Check sheet for the modelled part. Datum: model origin and axes. Units: mm. A direction names the side the tool comes from. Round coordinates to 2 decimals unless told otherwise and drop trailing zeros. Loops run counter-clockwise (first coordinate to the right, second up) from the corner with the lowest first, then second, coordinate; pieces in that order, holes last. Notation, with made-up numbers: (26, -3.5) -> (42, -3.5) arc R5 ccw to (42, 2.5) -> close; hole circle Ø6 at (77.25, -18). An arc over 180 degrees is marked (long way). Return JSON: item names as keys, results as strings.
from build123d import *

# Parameters (mm, degrees)
SKETCH1_W                                            = 40
SKETCH1_H                                            = 60
BOSS_EXTRUDE1_DEPTH                                  = 41
M2_5_CLEARANCE_HOLE1_D                               = 2.9
CUT_EXTRUDE1_DEPTH                                   = 33.5
FILLET1_R                                            = 1.6
F_16_0_16_DIAMETER_HOLE2_D                           = 16
SKETCH9_R                                            = 15.5
CUT_EXTRUDE2_DEPTH                                   = 33.5
FILLET2_R                                            = 4
CUT_EXTRUDE3_DEPTH                                   = 65.660652641
CUT_EXTRUDE3_DEPTH_BACK                              = 14
SKETCH11_W                                           = 50.653597067
SKETCH11_H                                           = 53.338920101
SKETCH12_R                                           = 15.5
CUT_EXTRUDE4_DEPTH                                   = 61.185131054
FILLET3_R                                            = 4
BOSS_EXTRUDE3_DEPTH                                  = 3
CHAMFER1_SIZE                                        = 6
BOSS_EXTRUDE4_DEPTH                                  = 41
CUT_EXTRUDE5_DEPTH                                   = 67.715815216
CUT_EXTRUDE5_DEPTH_BACK                              = 67.715815216
SKETCH19_W                                           = 48.667082547
SKETCH19_H                                           = 18.204733745
CBORE_FOR_M2_5_HEX_SOCKET_HEAD_CAP_SCREW_D           = 2.9
CBORE_FOR_M2_5_HEX_SOCKET_HEAD_CAP_SCREW_CBORE_D     = 5
CBORE_FOR_M2_5_HEX_SOCKET_HEAD_CAP_SCREW_CBORE_DEPTH = 20
TAP_DRILL_FOR_M3_HELICOIL1_D                         = 3.2
TAP_DRILL_FOR_M3_HELICOIL1_DEPTH                     = 4
TAP_DRILL_FOR_M3_HELICOIL1_TIP                       = 0.96137699
TAP_DRILL_FOR_M3_HELICOIL2_D                         = 3.15
TAP_DRILL_FOR_M3_HELICOIL2_DEPTH                     = 4.5
TAP_DRILL_FOR_M3_HELICOIL2_TIP                       = 0.946355475


with BuildPart() as part:
    # Sketch1 → Boss-Extrude1 (new body)
    with BuildSketch(Plane(origin=(0, 0, 0), x_dir=(1, 0, 0), z_dir=(0, 1, 0))):
        with Locations((-20, 0)):
            Rectangle(SKETCH1_W, SKETCH1_H)
    extrude(amount=BOSS_EXTRUDE1_DEPTH)

    # M2.5 Clearance Hole1 (through all)
    with Locations(Plane(origin=(0, 41, 0), x_dir=(1, 0, 0), z_dir=(0, 1, 0))):
        with Locations((-37.3, 26), (-37.3, 4), (-37.3, -18), (-31, -25.8), (-9, -25.8), (-2.7, -18), (-2.7, 4), (-2.7, 26)):
            Hole(M2_5_CLEARANCE_HOLE1_D / 2)

    # Sketch4 → Cut-Extrude1 (cut)
    with BuildSketch(Plane(origin=(0, 41, 0), x_dir=(1, 0, 0), z_dir=(0, 1, 0))):
        Polygon((-34.6, 30), (-34.6, -19), (-30, -19), (-30, -23), (-10, -23), (-10, -19), (-5.4, -19), (-5.4, 30), align=None)
    extrude(amount=-CUT_EXTRUDE1_DEPTH, mode=Mode.SUBTRACT)

    # Fillet1
    fillet1_edges = [part.edges().sort_by_distance(p)[0] for p in [
        (-10, 24.25, 23),
        (-30, 24.25, 23),
        (-30, 24.25, 19),
        (-34.6, 24.25, 19),
        (-5.4, 24.25, 19),
        (-10, 24.25, 19),
    ]]
    fillet(fillet1_edges, radius=FILLET1_R)

    # Ø16.0 (16) Diameter Hole2 (through all)
    with Locations(Plane(origin=(0, 7.5, 0), x_dir=(1, 0, 0), z_dir=(0, 1, 0))):
        with Locations((-20, -6)):
            Hole(F_16_0_16_DIAMETER_HOLE2_D / 2)

    # Sketch9 → Cut-Extrude2 (cut)
    with BuildSketch(Plane(origin=(0, 7.5, 0), x_dir=(1, 0, 0), z_dir=(0, 1, 0))):
        with Locations((-20, -6)):
            Circle(SKETCH9_R)
    extrude(amount=CUT_EXTRUDE2_DEPTH, mode=Mode.SUBTRACT)

    # Fillet2
    fillet2_edges = [part.edges().sort_by_distance(p)[0] for p in [
        (-5.4, 24.25, 0.795194528),
        (-5.4, 24.25, 11.204805472),
        (-34.6, 24.25, 11.204805472),
        (-34.6, 24.25, 0.795194528),
    ]]
    fillet(fillet2_edges, radius=FILLET2_R)

    # Sketch11 → Cut-Extrude3 (cut, two sides: drawn at the far end of the back side and taken through both)
    with BuildSketch(Plane(origin=(0, 41, 0), x_dir=(1, 0, 0), z_dir=(0, 1, 0)).offset(-CUT_EXTRUDE3_DEPTH_BACK)):
        with Locations((-19.614312713, -11.741576857)):
            Rectangle(SKETCH11_W, SKETCH11_H)
    extrude(amount=CUT_EXTRUDE3_DEPTH + CUT_EXTRUDE3_DEPTH_BACK, mode=Mode.SUBTRACT)

    # Sketch12 → Cut-Extrude4 (cut, through all)
    with BuildSketch(Plane(origin=(0, 7.5, 0), x_dir=(1, 0, 0), z_dir=(0, 1, 0))):
        with Locations((-20, 22)):
            Circle(SKETCH12_R)
    extrude(amount=CUT_EXTRUDE4_DEPTH, mode=Mode.SUBTRACT)

    # Fillet3
    fillet3_edges = [part.edges().sort_by_distance(p)[0] for p in [
        (-34.6, 24.25, -27.204805472),
        (-5.4, 24.25, -27.204805472),
        (-34.6, 24.25, -16.795194528),
        (-5.4, 24.25, -16.795194528),
    ]]
    fillet(fillet3_edges, radius=FILLET3_R)

    # Sketch15 → Boss-Extrude3 (add)
    with BuildSketch(Plane(origin=(0, 0, -30), x_dir=(-1, 0, 0), z_dir=(0, 0, -1))):
        Polygon((40, 41), (34.6, 41), (34.6, 7.5), (5.4, 7.5), (5.4, 41), (0, 41), (0, 0), (40, 0), align=None)
    extrude(amount=BOSS_EXTRUDE3_DEPTH)

    # Chamfer1
    chamfer1_edges = [part.edges().sort_by_distance(p)[0] for p in [
        (0, 13.5, 30),
        (-40, 13.5, 30),
    ]]
    chamfer(chamfer1_edges, length=CHAMFER1_SIZE)

    # Sketch18 → Boss-Extrude4 (add)
    with BuildSketch(Plane.XZ):
        Polygon((0, 24), (0, -33), (1, -33), (1, 24.414213562), (-5.585786438, 31), (-34.414213562, 31), (-41, 24.414213562), (-41, -33), (-40, -33), (-40, 24), (-34, 30), (-6, 30), align=None)
    extrude(amount=-BOSS_EXTRUDE4_DEPTH)

    # Sketch19 → Cut-Extrude5 (cut, two sides: drawn at the far end of the back side and taken through both)
    with BuildSketch(Plane.ZY.offset(-CUT_EXTRUDE5_DEPTH_BACK)):
        with Locations((9.40565808, 36.102366872)):
            Rectangle(SKETCH19_W, SKETCH19_H)
    extrude(amount=CUT_EXTRUDE5_DEPTH + CUT_EXTRUDE5_DEPTH_BACK, mode=Mode.SUBTRACT)

    # CBORE for M2.5 Hex Socket Head Cap Screw1 (through all)
    with Locations(Plane(origin=(0, 0, 0), x_dir=(-1, 0, 0), z_dir=(0, -1, 0))):
        with Locations((2.7, 4), (37.3, 4), (37.3, -18), (31, -25.8), (9, -25.8), (2.7, -18), (2.7, 26), (37.3, 26)):
            CounterBoreHole(CBORE_FOR_M2_5_HEX_SOCKET_HEAD_CAP_SCREW_D / 2, CBORE_FOR_M2_5_HEX_SOCKET_HEAD_CAP_SCREW_CBORE_D / 2, CBORE_FOR_M2_5_HEX_SOCKET_HEAD_CAP_SCREW_CBORE_DEPTH)

    # Tap Drill for M3 Helicoil1
    with Locations(Plane(origin=(0, 0, -33), x_dir=(-1, 0, 0), z_dir=(0, 0, -1))):
        with Locations((37.8, 35), (8, 3.75), (32, 3.75), (2.2, 35)):
            Hole(TAP_DRILL_FOR_M3_HELICOIL1_D / 2, depth=TAP_DRILL_FOR_M3_HELICOIL1_DEPTH)
            with Locations((0, 0, -(TAP_DRILL_FOR_M3_HELICOIL1_DEPTH + TAP_DRILL_FOR_M3_HELICOIL1_TIP / 2))):  # 118° drill point
                Cone(0, TAP_DRILL_FOR_M3_HELICOIL1_D / 2, TAP_DRILL_FOR_M3_HELICOIL1_TIP, mode=Mode.SUBTRACT)

    # Tap Drill for M3 Helicoil2
    with Locations(Plane.ZY.offset(41)):
        with Locations((7, 6.75), (7, 13.5), (7, 20.25), (-15, 6.75), (-15, 13.5), (-15, 20.25)):
            Hole(TAP_DRILL_FOR_M3_HELICOIL2_D / 2, depth=TAP_DRILL_FOR_M3_HELICOIL2_DEPTH)
            with Locations((0, 0, -(TAP_DRILL_FOR_M3_HELICOIL2_DEPTH + TAP_DRILL_FOR_M3_HELICOIL2_TIP / 2))):  # 118° drill point
                Cone(0, TAP_DRILL_FOR_M3_HELICOIL2_D / 2, TAP_DRILL_FOR_M3_HELICOIL2_TIP, mode=Mode.SUBTRACT)


solid = part.part
Q1. Section check A-A (x = -20). Record the boundary of the cut face in (y, z), then the cut area to 3 significant figures.
Results list:
{"outline": "(0, -33) -> (7.5, -33) -> (7.5, -2) -> (0, -2) -> close; (0, 14) -> (7.5, 14) -> (7.5, 23) -> (27, 23) -> (27, 31) -> (0, 31) -> close", "area": "516 mm^2"}
Q2. Material ranges on line 1 (X direction, y = 23, z = -11); line 2 (X direction, y = 2, z = -28); line 3 (Z direction, x = -2.7, y = 15), recorded low to high.
Results list:
{"line 1": "-41 to -34.6, -5.4 to 1", "line 2": "-41 to -38.8, -35.8 to -4.2, -1.2 to 1", "line 3": "-33 to -28.5, -23.5 to -6.5, -1.5 to 15.5, 20.5 to 28.11"}
Q3. Draft check along Z on faces 1 (the flat face through (-20, 17, 23)), 2 (the cylindrical face through (-38.718, 18.853, -15.727)), 3 (the flat face through (-5.4, 17, 15)). Enter one of: released by +Z, released by -Z, zero draft, split by the parting line, or undercut.
Results list:
{"face 1": "released by -Z", "face 2": "undercut", "face 3": "zero draft"}
Q4. Tool access check on faces 4 (the cylindrical face through (-30.46, 9.86, 28.24)), 5 (the cylindrical face through (-9.27, 2.78, -30.97)), 6 (the cylindrical face through (-35.5, 17.1, 5.9)), 7 (the cylindrical face through (-34.14, 17.11, 18.52)). Record the directions out of +Z, -Z, +X, -X, +Y, -Y that give a thin tool (end or side, any length) a straight path to the whole face; none if there is none.
Results list:
{"face 4": "-Y", "face 5": "-Z", "face 6": "+Y", "face 7": "-Z, +Y"}
Q5. Go/stop test with flat-tipped pins: pin 1 (1.5 mm diameter, centred on x = -28.5, z = -20.5, fed in from -Y); pin 2 (2.5 mm diameter, centred on x = -37.3, z = 18, fed in from +Y); pin 3 (18.5 mm diameter, centred on x = -23.5, y = 17, fed in from -Z); pin 4 (1.5 mm diameter, centred on x = -2, z = -3, fed in from -Y). Record where each tip stops, or that it passes through.
Results list:
{"pin 1": "y = 0", "pin 2": "through", "pin 3": "z = 19", "pin 4": "y = 20"}
Q6. Section check B-B (x = -14.5). Record the boundary of the cut face in (y, z).
Results list:
{"outline": "(0, -33) -> (7.5, -33) -> (7.5, 0.19) -> (0, 0.19) -> close; (0, 11.81) -> (7.5, 11.81) -> (7.5, 23) -> (27, 23) -> (27, 31) -> (0, 31) -> close"}
